```python
from build123d import *

# Parameters (mm, degrees)
F0_W        = 45
F0_H        = 36.6
F1_DEPTH    = 12.3
F2_W        = 37.3
F2_H        = 8.2
F3_DEPTH    = 36.601
F4_W        = 45
F4_H        = 16
F5_DEPTH    = 0.45
F6_T4_DEPTH = 47.571682988
F7_W        = 45
F7_H        = 4
F8_DEPTH    = 14.8
F9_R        = 3
F10_W       = 8.5
F10_H       = 4
F11_DEPTH   = 10.8
F12_R       = 3
F13_R       = 1.5
F14_DEPTH   = 25
F15_R       = 1.5
F16_DEPTH   = 25


# Not quite as in the source:
# - a fillet or chamfer that OpenCascade refuses, or shapes differently, is made with other operations: its cross-section is extruded or revolved along the edge and cut away or added


with BuildPart() as f1:
    # F0 (on Top) → F1 (new body)
    with BuildSketch(Plane.XY):
        Rectangle(F0_W, F0_H)
    extrude(amount=F1_DEPTH)

    # F2 (on face) → F3 (cut, through all)
    with BuildSketch(Plane.XZ.offset(18.3)):
        with Locations((0, 4.1)):
            Rectangle(F2_W, F2_H)
    extrude(amount=-F3_DEPTH, mode=Mode.SUBTRACT)

    # F4 (on face) → F5 (join)
    with BuildSketch(Plane.XY.offset(12.3)):
        with Locations((0, 10.3)):
            Rectangle(F4_W, F4_H)
    extrude(amount=F5_DEPTH)

    # F6: chamfer of 0.5 on 1 edges, made by hand


with BuildPart() as f6_tool2:
    # F6_s3 → F6_t4 (new body)
    with BuildSketch(Plane.YZ.offset(-23.785841494)):
        Polygon((2.3, 12.25), (2.8, 12.75), (2.3, 12.75), align=None)
    extrude(amount=F6_T4_DEPTH)

    split(bisect_by=Plane.XY.offset(12.3), keep=Keep.TOP)


with BuildPart() as f1_1:
    add(f1.part)

    # F6_t1: cut F6_tool2
    add(f6_tool2.part, mode=Mode.SUBTRACT)

    # F7 (on face) → F8 (join)
    with BuildSketch(Plane.XY.offset(12.75)):
        with Locations((0, 16.3)):
            Rectangle(F7_W, F7_H)
    extrude(amount=F8_DEPTH)

    # F9
    f9_edges = [f1_1.edges().sort_by_distance(p)[0] for p in [
        (-22.5, 16.3, 27.55),
        (22.5, 16.3, 27.55),
    ]]
    fillet(f9_edges, radius=F9_R)

    # F10 (on face) → F11 (join)
    with BuildSketch(Plane(origin=(0, 18.3, 0), x_dir=(-1, 0, 0), z_dir=(0, 1, 0))):
        with Locations((14.4, 10.2)):
            Rectangle(F10_W, F10_H)
    extrude(amount=F11_DEPTH)

    # F12
    f12_edges = [f1_1.edges().sort_by_distance(p)[0] for p in [
        (-10.15, 29.1, 10.2),
        (-18.65, 29.1, 10.2),
    ]]
    fillet(f12_edges, radius=F12_R)

    # F13 (on face) → F14 (cut)
    with BuildSketch(Plane.XY.offset(12.2)):
        with Locations((-14.4, 25.3)):
            Circle(F13_R)
        with Locations((-14.4, 20.3)):
            Circle(F13_R)
    extrude(amount=-F14_DEPTH, mode=Mode.SUBTRACT)

    # F15 (on face) → F16 (cut)
    with BuildSketch(Plane.XY.offset(12.75)):
        with Locations((-14.4, 5.2980469912)):
            Circle(F15_R)
    extrude(amount=-F16_DEPTH, mode=Mode.SUBTRACT)


solid = f1_1.part
```
The listing builds one solid part. Answer for the finished solid, in the listing's coordinates (mm). A direction names the side the tool comes from. Give positions to 0.01 mm unless a question says otherwise; leave off trailing zeros. Write each loop counter-clockwise with the first axis right and the second up, starting at its lowest first coordinate (ties: lowest second). Pieces come first, ordered by that corner, then holes. Notation, with made-up numbers: M 59,-8.75 L 102,-8.75 A19 cw 102,20.25 Z; hole C 77.25,-39.75 d5. An arc over 180 degrees is marked long. Write each question's results on one line, items separated by ' | '.
Q1. Section D-D, the plane x = 1 is taken. Write down the section's boundary in (y, z), then the cut area to 3 significant figures.
Output values:
outline: M -18.3,8.2 L 18.3,8.2 L 18.3,27.55 L 14.3,27.55 L 14.3,12.75 L 2.8,12.75 L 2.35,12.3 L -18.3,12.3 Z | area: 216 mm2
Q2. Section B-B, the plane x = -14.4 is taken. Write down the section's boundary in (y, z).
Output values:
outline: M -18.3,8.2 L 3.8,8.2 L 3.8,12.75 L 2.8,12.75 L 2.35,12.3 L -18.3,12.3 Z; M 6.8,8.2 L 18.8,8.2 L 18.8,12.2 L 18.3,12.2 L 18.3,27.55 L 14.3,27.55 L 14.3,12.75 L 6.8,12.75 Z; M 21.8,8.2 L 23.8,8.2 L 23.8,12.2 L 21.8,12.2 Z; M 26.8,8.2 L 29.1,8.2 L 29.1,12.2 L 26.8,12.2 Z
Q3. Flat-ended cylindrical pins translate along their axes: P1, Ø1.2, axis at y = 23, z = 10.5, coming from the +X side; P2, Ø1.8, axis at x = -14.4, y = 5.3, coming from the -Z side; P3, Ø11, axis at x = -1, y = 13, coming from the -Z side; P4, Ø6, axis at x = -6, z = 15, coming from the +Y side. Find the tip coordinate at first contact, or state that the pin passes through.
Output values:
P1: x = -10.15 | P2: through | P3: z = 8.2 | P4: y = 18.3
Q4. A tool of negligible diameter and unlimited length cuts with its end or side. For faces 5 (the flat face through (0, 9, 12.75)), 6 (the cylindrical face through (-17.75, 28.24, 10.23)), 7 (the flat face through (18.65, 0, 4)), from which of +Z, -Z, +X, -X, +Y, -Y can it reach the whole face along a straight path? Write none if from no direction.
Output values:
face 5: +Z, +X, -X, -Y | face 6: +Z, -Z, -X, +Y | face 7: -Z, +Y, -Y
Q5. Section C-C, the plane y = 25.3 is taken. Write down the section's boundary in (x, z), then the cut area to 3 significant figures.
Output values:
outline: M -18.65,8.2 L -15.9,8.2 L -15.9,12.2 L -18.65,12.2 Z; M -12.9,8.2 L -10.15,8.2 L -10.15,12.2 L -12.9,12.2 Z | area: 22.0 mm2
Q6. Consider L1, parallel to Y at x = -14.4, z = 9.45; L2, parallel to X at y = 3.5, z = 6.25; L3, parallel to Z at x = -19, y = -11.5. Determine where each line is inside the solid, lowest interval first. Write a range as from..to.
Output values:
L1: -18.3..3.8, 6.8..18.8, 21.8..23.8, 26.8..29.1 | L2: -22.5..-18.65, 18.65..22.5 | L3: 0..12.3
Q7. For a pull along X with two mould halves and no side action, classify faces 1 (the flat face through (-18.65, 0, 4)), 2 (the cylindrical face through (21.64, 16.33, 26.65)), 3 (the flat face through (0, 18.3, 17)), 4 (the flat face through (0, 0, 8.2)) as released by +X, released by -X, zero draft, split by the parting line, or undercut.
Output values:
face 1: undercut | face 2: released by +X | face 3: zero draft | face 4: undercut
Q8. Section A-A, the plane z = 6 is taken. Write down the section's boundary in (x, y).
Output values:
outline: M -22.5,-18.3 L -18.65,-18.3 L -18.65,18.3 L -22.5,18.3 Z; M 18.65,-18.3 L 22.5,-18.3 L 22.5,18.3 L 18.65,18.3 Z
